```python
from build123d import *

# Parameters (mm, degrees)
SKETCH1_R             = 20
BOSS_EXTRUDE1_DEPTH   = 25
SKETCH3_R             = 16.8
BOSS_EXTRUDE2_DEPTH   = 5
SKETCH4_R             = 4.1
CUT_EXTRUDE1_DEPTH    = 31
SKETCH6_R             = 2.1
CUT_EXTRUDE2_DEPTH    = 31
CHAMFER1_SIZE         = 1
CHAMFER1_SIZE2        = 0.363970234
CHAMFER1_PART_2_SIZE  = 1
CHAMFER1_PART_2_SIZE2 = 0.363970234
CHAMFER1_PART_3_SIZE  = 1
CHAMFER1_PART_3_SIZE2 = 0.363970234
CHAMFER1_PART_4_SIZE  = 1
CHAMFER1_PART_4_SIZE2 = 0.363970234
SKETCH7_R             = 4.1
CUT_EXTRUDE3_DEPTH    = 5
CHAMFER2_SIZE         = 0.5
CHAMFER2_SIZE2        = 1.37373871
SKETCH8_W             = 50
SKETCH8_H             = 50
SKETCH8_R             = 20
SKETCH8_R_2           = 1.5
BOSS_EXTRUDE3_DEPTH   = 6
CUT_EXTRUDE4_DEPTH    = 31.0000001
CHAMFER3_SIZE         = 0.5
CHAMFER3_SIZE2        = 1.37373871
CUT_EXTRUDE5_DEPTH    = 6.5
CHAMFER4_SIZE         = 1


with BuildPart() as part:
    # Sketch1 → Boss-Extrude1 (new body)
    with BuildSketch(Plane(origin=(0, 0, 0), x_dir=(1, 0, 0), z_dir=(0, 1, 0))):
        Circle(SKETCH1_R)
    extrude(amount=BOSS_EXTRUDE1_DEPTH)

    # Sketch3 → Boss-Extrude2 (add)
    with BuildSketch(Plane.XZ):
        Circle(SKETCH3_R)
    extrude(amount=BOSS_EXTRUDE2_DEPTH)

    # Sketch4 → Cut-Extrude1 (cut, through all)
    with BuildSketch(Plane(origin=(0, 25, 0), x_dir=(1, 0, 0), z_dir=(0, 1, 0))):
        with Locations((8, 0)):
            Circle(SKETCH4_R)
        with Locations((-8, 0)):
            Circle(SKETCH4_R)
    extrude(amount=-CUT_EXTRUDE1_DEPTH, mode=Mode.SUBTRACT)

    # Sketch6 → Cut-Extrude2 (cut, through all)
    with BuildSketch(Plane(origin=(0, 25, 0), x_dir=(1, 0, 0), z_dir=(0, 1, 0))):
        with Locations((10.5, -10.5)):
            Circle(SKETCH6_R)
        with Locations((-10.5, -10.5)):
            Circle(SKETCH6_R)
        with Locations((-10.5, 10.5)):
            Circle(SKETCH6_R)
        with Locations((10.5, 10.5)):
            Circle(SKETCH6_R)
    extrude(amount=-CUT_EXTRUDE2_DEPTH, mode=Mode.SUBTRACT)

    # Chamfer1
    chamfer1_edges = [part.edges().sort_by_distance(p)[0] for p in [
        (0, -5, 16.8),
    ]]
    chamfer1_side = [part.faces().sort_by_distance(p)[0] for p in [
        (0, -2.5, 16.8),
    ]]
    chamfer(chamfer1_edges, length=CHAMFER1_SIZE, length2=CHAMFER1_SIZE2, reference=chamfer1_side[0])

    # Chamfer1 part 2
    chamfer1_part_2_edges = [part.edges().sort_by_distance(p)[0] for p in [
        (-16.8, -5, 0),
    ]]
    chamfer1_part_2_side = [part.faces().sort_by_distance(p)[0] for p in [
        (-16.8, -2.5, 0),
    ]]
    chamfer(chamfer1_part_2_edges, length=CHAMFER1_PART_2_SIZE, length2=CHAMFER1_PART_2_SIZE2, reference=chamfer1_part_2_side[0])

    # Chamfer1 part 3
    chamfer1_part_3_edges = [part.edges().sort_by_distance(p)[0] for p in [
        (0, -5, -16.8),
    ]]
    chamfer1_part_3_side = [part.faces().sort_by_distance(p)[0] for p in [
        (0, -2.5, -16.8),
    ]]
    chamfer(chamfer1_part_3_edges, length=CHAMFER1_PART_3_SIZE, length2=CHAMFER1_PART_3_SIZE2, reference=chamfer1_part_3_side[0])

    # Chamfer1 part 4
    chamfer1_part_4_edges = [part.edges().sort_by_distance(p)[0] for p in [
        (16.8, -5, 0),
    ]]
    chamfer1_part_4_side = [part.faces().sort_by_distance(p)[0] for p in [
        (16.8, -2.5, 0),
    ]]
    chamfer(chamfer1_part_4_edges, length=CHAMFER1_PART_4_SIZE, length2=CHAMFER1_PART_4_SIZE2, reference=chamfer1_part_4_side[0])

    # Sketch7 → Cut-Extrude3 (cut)
    with BuildSketch(Plane(origin=(0, 25, 0), x_dir=(1, 0, 0), z_dir=(0, 1, 0))):
        with Locations((10.5, 10.5)):
            Circle(SKETCH7_R)
        with Locations((-10.5, 10.5)):
            Circle(SKETCH7_R)
        with Locations((-10.5, -10.5)):
            Circle(SKETCH7_R)
        with Locations((10.5, -10.5)):
            Circle(SKETCH7_R)
    extrude(amount=-CUT_EXTRUDE3_DEPTH, mode=Mode.SUBTRACT)

    # Chamfer2
    chamfer2_edges = [part.edges().sort_by_distance(p)[0] for p in [
        (3.9, 25, 0),
    ]]
    chamfer2_side = [part.faces().sort_by_distance(p)[0] for p in [
        (0, 25, 0),
    ]]
    chamfer(chamfer2_edges, length=CHAMFER2_SIZE, length2=CHAMFER2_SIZE2, reference=chamfer2_side[0])

    # Sketch8 → Boss-Extrude3 (add)
    with BuildSketch(Plane(origin=(0, 25, 0), x_dir=(1, 0, 0), z_dir=(0, 1, 0))):
        Rectangle(SKETCH8_W, SKETCH8_H)
        Circle(SKETCH8_R, mode=Mode.SUBTRACT)
        with Locations((-16.617009358, -16.617009358)):
            Circle(SKETCH8_R_2, mode=Mode.SUBTRACT)
        with Locations((-16.617009358, 16.617009358)):
            Circle(SKETCH8_R_2, mode=Mode.SUBTRACT)
        with Locations((16.617009358, 16.617009358)):
            Circle(SKETCH8_R_2, mode=Mode.SUBTRACT)
        with Locations((16.617009358, -16.617009358)):
            Circle(SKETCH8_R_2, mode=Mode.SUBTRACT)
    extrude(amount=-BOSS_EXTRUDE3_DEPTH)

    # Sketch10 → Cut-Extrude4 (cut, through all)
    with BuildSketch(Plane(origin=(0, 25, 0), x_dir=(1, 0, 0), z_dir=(0, 1, 0))):
        Polygon((-19.975766569, -18.915106397), (-18.915106397, -19.975766569), (-23.939339828, -25), (-25, -25), (-25, -23.939339828), align=None)
        Polygon((-25, 23.939339828), (-19.975766569, 18.915106397), (-18.915106397, 19.975766569), (-23.939339828, 25), (-25, 25), align=None)
        Polygon((23.939339828, 25), (18.915106397, 19.975766569), (19.975766569, 18.915106397), (25, 23.939339828), (25, 25), align=None)
        Polygon((18.915106397, -19.975766569), (19.975766569, -18.915106397), (25, -23.939339828), (25, -25), (23.939339828, -25), align=None)
    extrude(amount=-CUT_EXTRUDE4_DEPTH, mode=Mode.SUBTRACT)

    # Chamfer3
    chamfer3_edges = [part.edges().sort_by_distance(p)[0] for p in [
        (6.4, 25, -10.5),
        (-14.6, 25, -10.5),
        (-14.6, 25, 10.5),
        (6.4, 25, 10.5),
    ]]
    chamfer3_side = [part.faces().sort_by_distance(p)[0] for p in [
        (-0.052152151, 25, 0),
    ]]
    chamfer(chamfer3_edges, length=CHAMFER3_SIZE, length2=CHAMFER3_SIZE2, reference=chamfer3_side[0])

    # Sketch11 → Cut-Extrude5 (cut)
    with BuildSketch(Plane.XZ.offset(5)):
        Polygon((-8, 7.5), (-14.495190528, 3.75), (-14.495190528, -3.75), (-8, -7.5), (-1.504809472, -3.75), (-1.504809472, 3.75), align=None)
        Polygon((8, 7.5), (1.504809472, 3.75), (1.504809472, -3.75), (8, -7.5), (14.495190528, -3.75), (14.495190528, 3.75), align=None)
    extrude(amount=-CUT_EXTRUDE5_DEPTH, mode=Mode.SUBTRACT)

    # Chamfer4
    chamfer4_edges = [part.edges().sort_by_distance(p)[0] for p in [
        (-20, 19, 0),
        (-4.752404736, -5, 5.625),
        (-11.247595264, -5, 5.625),
        (-14.495190528, -5, 0),
        (-11.247595264, -5, -5.625),
        (-4.752404736, -5, -5.625),
        (-1.504809472, -5, 0),
        (11.247595264, -5, 5.625),
        (4.752404736, -5, 5.625),
        (1.504809472, -5, 0),
        (4.752404736, -5, -5.625),
        (11.247595264, -5, -5.625),
        (14.495190528, -5, 0),
    ]]
    chamfer(chamfer4_edges, length=CHAMFER4_SIZE)


solid = part.part
```
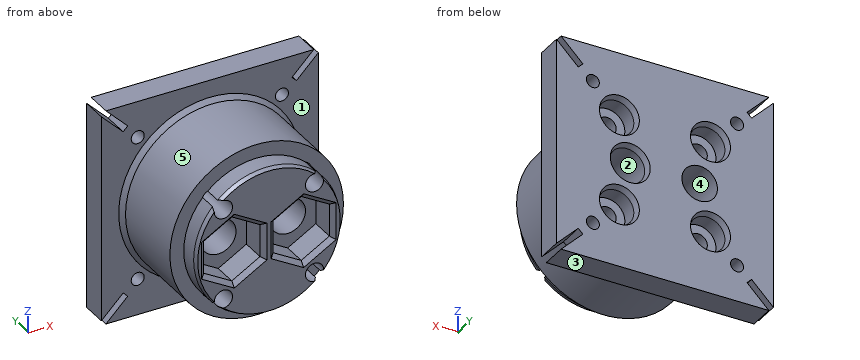
Part model, mm, in its own coordinate system. Face numbers are marked on the shaded views. A direction names the side the tool comes from. Coordinates: 2 decimals unless noted, no trailing zeros. Order: outer loops, then holes, each group sorted by start corner. A loop starts at its lowest first (then second) coordinate and runs counter-clockwise, first axis right, second up. Notation, with made-up numbers: (55.5, 31) - (88.5, 31) arc R20 ccw to (88.5, 35) - close; hole circle Ø11 at (-27.5, 84). An arc over 180 degrees is marked (long way). Return JSON: item names as keys, results as strings. Group by question number.
Item 1: Which spindle directions (+Z, -Z, +X, -X, +Y, -Y) get a long thin tool onto all of the face, cutting with end or side? Do the marked faces 4 and 5. Say none if no direction does.
Item 2: Cut at C-C (x = 17.5). State how many separate pieces and enclosed holes the cut face has, plus the area to 3 significant figures.
Item 3: Pull direction Z, two halves, no side cores. Call the marked faces 1, 2 and 3: pulls with the +Z half, pulls with the -Z half, needs draft (parallel to the pull), parting line crosses it, or undercut.
Item 4: Pin check, flat tips, straight feed: pin 1 (3 mm diameter, centred on y = 10.5, z = 2, fed in from +X); pin 2 (5 mm diameter, centred on x = 10.5, z = 10.5, fed in from +Y); pin 3 (6.5 mm diameter, centred on x = -8, z = 1, fed in from -Y). Stop position of each tip, or through.
Item 5: Cut at B-B (z = 22.5). List the corners of the cut face in (x, y), plus the area to 3 significant figures.
Item 6: Cut at A-A (y = 7). List the corners of the cut face in (x, z), plus the area to 3 significant figures.
Item 7: Drill centre lines: probe 1 along X at (y, z) = (21, -10); probe 2 along Z at (x, y) = (10.5, 22.2); probe 3 along X at (y, z) = (5, 2.5). Where is each one in solid material? Low to high. Write a range as from..to.
Check values:
{
 "1": {"face 4": "+Y, -Y", "face 5": "-Y"},
 "2": {"separate pieces": "3", "enclosed holes": "0", "area": "641 mm2"},
 "3": {"face 1": "needs draft", "face 2": "undercut", "face 3": "pulls with the -Z half"},
 "4": {"pin 1": "stops at x = 19.99", "pin 2": "stops at y = 20", "pin 3": "stops at y = 1.5"},
 "5": {"outline": "(-25, 19) - (-23.56, 19) - (-23.56, 25) - (-25, 25) - close; (-21.44, 19) - (21.44, 19) - (21.44, 25) - (-21.44, 25) - close; (23.56, 19) - (25, 19) - (25, 25) - (23.56, 25) - close", "area": "275 mm2"},
 "6": {"outline": "circle Ø40 at (0, 0); hole circle Ø4.2 at (-10.5, -10.5); hole circle Ø4.2 at (-10.5, 10.5); hole circle Ø8.2 at (-8, 0); hole circle Ø8.2 at (8, 0); hole circle Ø4.2 at (10.5, -10.5); hole circle Ø4.2 at (10.5, 10.5)", "area": "1,100 mm2"},
 "7": {"probe 1": "x = -25..-14.57, -6.43..6.43, 14.57..25", "probe 2": "z = -25..-14.6, -6.4..-3.25, 3.25..6.4, 14.6..25", "probe 3": "x = -19.84..-11.25, -4.75..4.75, 11.25..19.84"}
}
